from build123d import *

# Parameters (mm, degrees)
PAD_DEPTH       = 26
SKETCH001_R     = 2
POCKET_DEPTH    = 4
SKETCH002_R     = 3.3
POCKET001_DEPTH = 4
FILLET_R        = 2
FILLET001_R     = 2
FILLET002_R     = 2


with BuildPart() as part:
    # Sketch → Pad (new body)
    with BuildSketch(Plane.XY):
        Polygon((0, 0), (0, 52), (22, 52), (22, 48), (4, 48), (4, 0), align=None)
    extrude(amount=PAD_DEPTH)

    # Sketch001 (on Face2 of Pad) → Pocket (cut)
    with BuildSketch(Plane(origin=(0, 52, 0), x_dir=(-1, 0, 0), z_dir=(0, 1, 0))):
        with Locations((-19, 3)):
            Circle(SKETCH001_R)
        with Locations((-19, 23)):
            Circle(SKETCH001_R)
    extrude(amount=-POCKET_DEPTH, mode=Mode.SUBTRACT)

    # Sketch002 (on Face1 of Pocket) → Pocket001 (cut)
    with BuildSketch(Plane(origin=(0, 0, 0), x_dir=(0, -1, 0), z_dir=(-1, 0, 0))):
        with Locations((-10, 13)):
            Circle(SKETCH002_R)
        with BuildLine():
            ThreePointArc((-27, 16.3), (-30.3, 13), (-27, 9.7))
            Line((-27, 9.7), (-20, 9.7))
            ThreePointArc((-20, 9.7), (-16.7, 13), (-20, 16.3))
            Line((-27, 16.3), (-20, 16.3))
        make_face()
        with BuildLine():
            ThreePointArc((-44, 16.3), (-47.3, 13), (-44, 9.7))
            Line((-44, 9.7), (-37, 9.7))
            ThreePointArc((-37, 9.7), (-33.7, 13), (-37, 16.3))
            Line((-44, 16.3), (-37, 16.3))
        make_face()
    extrude(amount=-POCKET001_DEPTH, mode=Mode.SUBTRACT)

    # Fillet
    fillet_edges = [part.edges().sort_by_distance(p)[0] for p in [
        (0, 52, 13),
    ]]
    fillet(fillet_edges, radius=FILLET_R)

    # Fillet001
    fillet001_edges = [part.edges().sort_by_distance(p)[0] for p in [
        (2, 0, 0),
    ]]
    fillet(fillet001_edges, radius=FILLET001_R)

    # Fillet002
    fillet002_edges = [part.edges().sort_by_distance(p)[0] for p in [
        (2, 0, 26),
    ]]
    fillet(fillet002_edges, radius=FILLET002_R)


solid = part.part
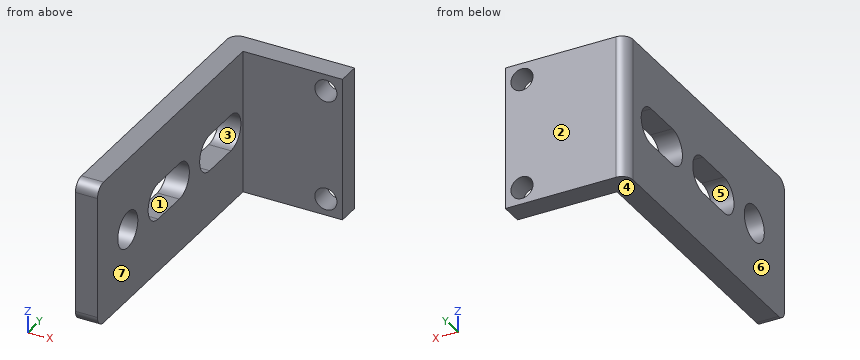
Read the model definition and answer for the solid it produces. Units are mm, in the model's axes. Face numbers are marked on the shaded views. A direction names the side the tool comes from. Round coordinates to 2 decimals unless told otherwise and drop trailing zeros. Loops run counter-clockwise (first coordinate to the right, second up) from the corner with the lowest first, then second, coordinate; pieces in that order, holes last. Notation, with made-up numbers: (52.25, 67.25) - (62.25, 67.25) arc R20 ccw to (62.25, 91.25) - close; hole circle Ø3 at (35, 57.5). An arc over 180 degrees is marked (long way). One line per question, with ' | ' between items. Start each with the question number.
Q1. Section B-B on z = 3 is taken. Give the vertices of the cut face in (x, y), plus the area to 3 significant figures.
Q2. Section D-D on z = 19.5 is taken. Give the vertices of the cut face in (x, y).
Q3. For a pull along Y with two mould halves and no side action, classify the marked faces 1, 2, 3 and 4 as +Y half, -Y half, draft (parallel to the pull), parting line (faces both ways), or undercut.
Q4. Find the intervals of material crossed by L1, parallel to Z at x = 19, y = 49.5; L2, parallel to Z at x = 1.4, y = 10; L3, parallel to Y at x = 7, z = 14.25, in increasing order.
Q5. Section C-C on x = 19 is taken. Give the vertices of the cut face in (y, z).
Q6. Flat-ended cylindrical pins translate along their axes: pin 1 (4.5 mm diameter, centred on x = 19, z = 23, fed in from +Y); pin 2 (10 mm diameter, centred on y = 12.5, z = 13.5, fed in from +X); pin 3 (10 mm diameter, centred on x = 12, z = 17, fed in from -Y); pin 4 (3 mm diameter, centred on x = 19, z = 3, fed in from -Y). Find the tip coordinate at first contact, or state that the pin passes through.
Q7. Section A-A on y = 10 is taken. Give the vertices of the cut face in (x, z), plus the area to 3 significant figures.
Q8. For the marked faces 5, 6 and 7, determine the directions among +Z, -Z, +X, -X, +Y, -Y from which every point of the face is accessible in a straight line to the end or side of a thin tool.
Established:
1) outline: (0, 0) - (4, 0) - (4, 48) - (17, 48) - (17, 52) - (2, 52) arc R2 ccw to (0, 50) - close; (21, 48) - (22, 48) - (22, 52) - (21, 52) - close | area: 263 mm²
2) outline: (0, 0) - (4, 0) - (4, 48) - (22, 48) - (22, 52) - (2, 52) arc R2 ccw to (0, 50) - close
3) face 1: undercut | face 2: +Y half | face 3: undercut | face 4: draft
4) L1: 0 to 1, 5 to 21, 25 to 26 | L2: 0 to 9.7, 16.3 to 26 | L3: 48 to 52
5) outline: (48, 0) - (52, 0) - (52, 1) - (48, 1) - close; (48, 5) - (52, 5) - (52, 21) - (48, 21) - close; (48, 25) - (52, 25) - (52, 26) - (48, 26) - close
6) pin 1: y = 52 | pin 2: x = 4 | pin 3: y = 48 | pin 4: through
7) outline: (0, 0) - (4, 0) - (4, 9.7) - (0, 9.7) - close; (0, 16.3) - (4, 16.3) - (4, 26) - (0, 26) - close | area: 77.6 mm²
8) face 5: +X, -X | face 6: +Z, -Z, -X, +Y, -Y | face 7: +Z, -Z, +X, -Y
